Build history of the part. All positions in model axes, mm. Give positions to 0.01 mm unless a question says otherwise; leave off trailing zeros. Order: outer loops, then holes, each group sorted by start corner. A loop starts at its lowest first (then second) coordinate and runs counter-clockwise, first axis right, second up. Notation, with made-up numbers: (87, 50.5) -> (141, 50.5) arc R20 ccw to (141, 58.5) -> close; hole circle Ø8 at (0, -34). An arc over 180 degrees is marked (long way). Use a Markdown table: item, result. Add a question column.
```python
from build123d import *

# Parameters (mm, degrees)
BOSS_EXTRUDE1_DEPTH = 4
FILLET1_R           = 20
SKETCH1_R           = 10
SKETCH1_R_2         = 2.25
CUT_EXTRUDE3_DEPTH  = 131.855321132


with BuildPart() as part:
    # Sketch3 → Boss-Extrude1 (new body)
    with BuildSketch(Plane(origin=(0, 0, 0), x_dir=(1, 0, 0), z_dir=(0, 1, 0))):
        with BuildLine():
            Line((22.912878475, 10), (53.225121597, 8.941473145))
            ThreePointArc((53.225121597, 8.941473145), (61.859801844, 0), (53.225121597, -8.941473145))
            Line((53.225121597, -8.941473145), (22.912878475, -10))
            ThreePointArc((22.912878475, -10), (-25, 0), (22.912878475, 10))
        make_face()
    extrude(amount=BOSS_EXTRUDE1_DEPTH)

    # Fillet1
    fillet1_edges = [part.edges().sort_by_distance(p)[0] for p in [
        (22.912878475, 2, -10),
        (22.912878475, 2, 10),
    ]]
    fillet(fillet1_edges, radius=FILLET1_R)

    # Sketch1 → Cut-Extrude3 (cut, through all)
    with BuildSketch(Plane(origin=(103.38268991, 0, 0), x_dir=(1, 0, 0), z_dir=(0, 1, 0))):
        with Locations(Location((-103.38268991, 0, 0), (0, 0, 270))):
            Circle(SKETCH1_R)
        with Locations(Location((-103.38268991, 14.5, 0), (0, 0, 270))):
            Circle(SKETCH1_R_2)
        with Locations(Location((-76.469811435, 0, 0), (0, 0, 90))):
            Circle(SKETCH1_R_2)
        with Locations(Location((-50.469811435, 0, 0), (0, 0, 90))):
            Circle(SKETCH1_R_2)
        with Locations(Location((-103.38268991, -14.5, 0), (0, 0, 270))):
            Circle(SKETCH1_R_2)
    extrude(amount=CUT_EXTRUDE3_DEPTH, mode=Mode.SUBTRACT)


solid = part.part
```
(1) Band-saw the part on A-A on z = 0. Give the cut face in (x, y).
(2) Wall check: probe 1 along Z at (x, y) = (0, 0.3); probe 2 along X at (y, z) = (2.95, 0); probe 3 along X at (y, z) = (2.4, -16). Give the ranges that are in metal, low to high.
(3) Mould opens along X. For faces 1 (the face through (9, 0, -6)), 2 (the face through (25.39, 2.028, 11.516)), 3 (the face through (24.68, 1.97, 0.29)) say: released by +X, released by -X, zero draft, split by the parting line, or undercut.
(4) Band-saw the part on C-C on z = -14.5. Give the cut face in (x, y).
(5) Pin check, flat tips, straight feed: pin 1 Ø1.5 at (y, z) = (3.5, -3.5) entering from -X; pin 2 Ø2 at (x, y) = (28.5, 2) entering from +Z. Stop position of each tip, or through.
(6) Band-saw the part on D-D on y = 3. Give the cut face in (x, z).
(7) Band-saw the part on B-B on x = 0. Give the cut face in (y, z).
Response:
| question | item | result |
|---|---|---|
| 1 | outline | (-25, 0) -> (-10, 0) -> (-10, 4) -> (-25, 4) -> close; (10, 0) -> (24.66, 0) -> (24.66, 4) -> (10, 4) -> close; (29.16, 0) -> (50.66, 0) -> (50.66, 4) -> (29.16, 4) -> close; (55.16, 0) -> (61.86, 0) -> (61.86, 4) -> (55.16, 4) -> close |
| 2 | probe 1 | z = -25 to -16.75, -12.25 to -10, 10 to 12.25, 16.75 to 25 |
| 2 | probe 2 | x = -25 to -10, 10 to 24.66, 29.16 to 50.66, 55.16 to 61.86 |
| 2 | probe 3 | x = -19.21 to -1.68, 1.68 to 19.23 |
| 3 | face 1 | zero draft |
| 3 | face 2 | released by +X |
| 3 | face 3 | undercut |
| 4 | outline | (-20.37, 0) -> (-2.25, 0) -> (-2.25, 4) -> (-20.37, 4) -> close; (2.25, 0) -> (20.79, 0) -> (20.79, 4) -> (2.25, 4) -> close |
| 5 | pin 1 | stops at x = -24.85 |
| 5 | pin 2 | stops at z = 10.67 |
| 6 | outline | (18.82, -16.46) arc R20 cw to (33.17, -9.64) -> (53.23, -8.94) arc R8.95 ccw to (53.23, 8.94) -> (33.17, 9.64) arc R20 cw to (18.82, 16.46) arc R25 ccw (long way) to start; hole circle Ø20 at (0, 0); hole circle Ø4.5 at (0, -14.5); hole circle Ø4.5 at (0, 14.5); hole circle Ø4.5 at (26.91, 0); hole circle Ø4.5 at (52.91, 0) |
| 7 | outline | (0, -25) -> (4, -25) -> (4, -16.75) -> (0, -16.75) -> close; (0, -12.25) -> (4, -12.25) -> (4, -10) -> (0, -10) -> close; (0, 10) -> (4, 10) -> (4, 12.25) -> (0, 12.25) -> close; (0, 16.75) -> (4, 16.75) -> (4, 25) -> (0, 25) -> close |
